Build history of the part. All positions in model axes, mm. A direction names the side the tool comes from. Round coordinates to 2 decimals unless told otherwise and drop trailing zeros. Loops run counter-clockwise (first coordinate to the right, second up) from the corner with the lowest first, then second, coordinate; pieces in that order, holes last. Notation, with made-up numbers: (79, 32) - (107, 32) arc R11 ccw to (107, 52) - close; hole circle Ø1 at (12, 16.25). An arc over 180 degrees is marked (long way). Use one line per item in the form item = value. Start each with the question number.
Q1. Saw through at B-B (x = -2.25). Give the cut face in (y, z), then the cut area to 3 significant figures.
Q2. Saw through at C-C (y = 16.5). Give the cut face in (x, z), then the cut area to 3 significant figures.
Q3. Pin check, flat tips, straight feed: pin 1 (3 mm diameter, centred on x = -4, y = 25.5, fed in from +Z); pin 2 (3 mm diameter, centred on y = 22.5, z = -1, fed in from +X); pin 3 (1 mm diameter, centred on x = -1, z = 6.5, fed in from +Y); pin 4 (1.5 mm diameter, centred on y = 23.5, z = 5, fed in from -X). Stop position of each tip, or through.
Q4. 3-axis set-ups, long thin cutter, end or side, ignore diameter. For faces 1 (the face through (-3, 0, 2)), 2 (the face through (0, 13.9, 2)): which of +Z, -Z, +X, -X, +Y, -Y reach the whole face in a straight line?
Q5. Saw through at A-A (z = 1.25). Give the cut face in (x, y).
Q6. Saw through at D-D (z = -1). Give the cut face in (x, y), then the cut area to 3 significant figures.
Q7. Drill centre lines: line 1 (Y direction, x = -4.25, z = 5.25); line 2 (Y direction, x = -4, z = 4.75); line 3 (Z direction, x = -3.25, y = 20). Where is each one in solid material? Low to high.
Autodesk Inventor part; units mm, degrees
ref_plane "YZ Plane" through (0, 0, 0) normal (1, 0, 0) x (0, 1, 0)
ref_plane "XZ Plane" through (0, 0, 0) normal (0, 1, 0) x (-1, 0, 0)
ref_plane "XY Plane" through (0, 0, 0) normal (0, 0, 1) x (1, 0, 0)
sketch "Sketch1" plane through (0, 0, 0) normal (0, 1, 0) x (-1, 0, 0)
  line L0 (6.4234, 8.5987) -> (-0.2766, 8.5987)
  line L1 (-0.2766, 8.5987) -> (-0.2766, -4.1013)
  line L2 (-0.2766, -4.1013) -> (6.4234, -4.1013)
  line L3 (6.4234, -4.1013) -> (6.4234, 8.5987)
  point P0 (0, 0)
  dimension "d0" = 6.7
  dimension "d1" = 12.7
extrude "Extrusion1" add sketch "Sketch1" along normal blind 13.9
sketch "Sketch2" plane through (0, 13.9, 0) normal (0, 1, 0) x (1, 0, 0)
  circle A0 centre (-3.0734, -2.2487) radius 2.93
  point P0 (0, 0)
  point P1 (-6.4234, -8.5987)
  point P2 (0.2766, -8.5987)
  point P3 (-6.4234, 4.1013)
  dimension "d4" = 5.86
extrude "Extrusion2" add sketch "Sketch2" along normal blind 8.8
sketch "Sketch3" plane through (-3.0734, 22.7, 2.2487) normal (0, 1, 0) x (1, 0, 0)
  circle A0 centre (0, 0) radius 1.3
  point P0 (3.0734, 2.2487)
  dimension "d7" = 2.6
extrude "Extrusion3" add sketch "Sketch3" along normal blind 10.1
properties part number "Switch"
Report:
q1.outline = (0, -4.1) - (13.9, -4.1) - (13.9, -0.56) - (22.7, -0.56) - (22.7, 1.24) - (32.8, 1.24) - (32.8, 3.25) - (22.7, 3.25) - (22.7, 5.06) - (13.9, 5.06) - (13.9, 8.6) - (0, 8.6) - close
q1.area = 246 mm²
q2.outline = circle Ø5.86 at (-3.07, 2.25)
q2.area = 27.0 mm²
q3.pin_1 = 3.55
q3.pin_2 = -0.72
q3.pin_3 = 13.9
q3.pin_4 = through
q4.face_1 = +Z, -Z, +X, -X, -Y
q4.face_2 = +Y
q5.outline = (-6.42, 0) - (0.28, 0) - (0.28, 13.9) - (-0.32, 13.9) - (-0.32, 22.7) - (-2.24, 22.7) - (-2.24, 32.8) - (-3.91, 32.8) - (-3.91, 22.7) - (-5.83, 22.7) - (-5.83, 13.9) - (-6.42, 13.9) - close
q6.outline = (-6.42, 0) - (0.28, 0) - (0.28, 13.9) - (-6.42, 13.9) - close
q6.area = 93.1 mm²
q7.line_1 = 0 to 13.9
q7.line_2 = 0 to 22.7
q7.line_3 = -0.68 to 5.17
